Build history of the part. All positions in model axes, mm. A direction names the side the tool comes from. Coordinates: 2 decimals unless noted, no trailing zeros. Loops run counter-clockwise (first coordinate to the right, second up) from the corner with the lowest first, then second, coordinate; pieces in that order, holes last. Notation, with made-up numbers: (0, 89) - (57, 89) arc R16 cw to (57, 118) - close; hole circle Ø3 at (-22.75, 84.25). An arc over 180 degrees is marked (long way). One line per item, written item: value.
```python
from build123d import *

# Parameters (mm, degrees)
F1_DEPTH = 6.096
F3_DEPTH = 5.08
F4_W     = 19.05
F4_H     = 19.05
F5_DEPTH = 1.8542


with BuildPart() as f1:
    # F0 (on Top) → F1 (new body)
    with BuildSketch(Plane.XY):
        with BuildLine():
            ThreePointArc((0, 1.27), (0.371974, 0.371974), (1.27, 0))
            Line((1.27, 0), (15.24, 0))
            ThreePointArc((15.24, 0), (16.138026, 0.371974), (16.51, 1.27))
            Line((16.51, 1.27), (16.51, 15.24))
            ThreePointArc((16.51, 15.24), (16.138026, 16.138026), (15.24, 16.51))
            Line((15.24, 16.51), (1.27, 16.51))
            ThreePointArc((1.27, 16.51), (0.371974, 16.138026), (0, 15.24))
            Line((0, 15.24), (0, 1.27))
        make_face()
    extrude(amount=-F1_DEPTH)

    # F2 (on face) → F3 (cut)
    with BuildSketch(Plane(origin=(0, 0, -6.096), x_dir=(1, 0, 0), z_dir=(0, 0, -1))):
        with BuildLine():
            Line((13.97, -1.27), (2.54, -1.27))
            ThreePointArc((2.54, -1.27), (1.641974, -1.641974), (1.27, -2.54))
            Line((1.27, -2.54), (1.27, -13.97))
            ThreePointArc((1.27, -13.97), (1.641974, -14.868026), (2.54, -15.24))
            Line((2.54, -15.24), (13.97, -15.24))
            ThreePointArc((13.97, -15.24), (14.868026, -14.868026), (15.24, -13.97))
            Line((15.24, -13.97), (15.24, -2.54))
            ThreePointArc((15.24, -2.54), (14.868026, -1.641974), (13.97, -1.27))
        make_face()
    extrude(amount=-F3_DEPTH, mode=Mode.SUBTRACT)

    # F4 (on Top) → F5 (join)
    with BuildSketch(Plane.XY):
        with Locations((8.255, 8.255)):
            Rectangle(F4_W, F4_H)
    extrude(amount=F5_DEPTH)


solid = f1.part
```
Item 1: Tool access for faces 1 (the face through (0.382, 16.148, -3.005)), 2 (the face through (1.652, 1.632, -3.592)), 3 (the face through (16.148, 16.128, -3.005)): list every direction of +Z, -Z, +X, -X, +Y, -Y with a clear straight run to the whole face (end or side of a thin tool).
Check result:
face 1: -Z, -X, +Y
face 2: -Z
face 3: -Z, +X, +Y
Item 2: Drop flat-ended pins along their axis: P1, Ø2, axis at x = 13, z = -3, coming from the +Y side; P2, Ø3, axis at x = 11, z = -4.5, coming from the -Y side; P3, Ø4, axis at x = 9.5, y = 4, coming from the -Z side. Give the stop position or say it passes through.
Check result:
P1: stops at y = 16.51
P2: stops at y = 0
P3: stops at z = -1.02
Item 3: Cut at A-A, the plane z = -4.25. Write the cut outline in (x, y), then the cut area to 3 significant figures.
Check result:
outline: (0, 1.27) arc R1.27 ccw to (1.27, 0) - (15.24, 0) arc R1.27 ccw to (16.51, 1.27) - (16.51, 15.24) arc R1.27 ccw to (15.24, 16.51) - (1.27, 16.51) arc R1.27 ccw to (0, 15.24) - close; hole (1.27, 2.54) arc R1.27 ccw to (2.54, 1.27) - (13.97, 1.27) arc R1.27 ccw to (15.24, 2.54) - (15.24, 13.97) arc R1.27 ccw to (13.97, 15.24) - (2.54, 15.24) arc R1.27 ccw to (1.27, 13.97) - close
area: 77.4 mm^2
Item 4: Cut at B-B, the plane x = 11.75. Write the cut outline in (y, z), then the cut area to 3 significant figures.
Check result:
outline: (-1.27, 0) - (0, 0) - (0, -6.1) - (1.27, -6.1) - (1.27, -1.02) - (15.24, -1.02) - (15.24, -6.1) - (16.51, -6.1) - (16.51, 0) - (17.78, 0) - (17.78, 1.85) - (-1.27, 1.85) - close
area: 65.0 mm^2
Item 5: Probe probe 1 along Y at (x, z) = (4.5, -2.5); probe 2 along Z at (x, y) = (5.25, 6). List the from-to ranges inside material, lowest first. Write a range as from..to.
Check result:
probe 1: y = 0..1.27, 15.24..16.51
probe 2: z = -1.02..1.85
Item 6: Pull direction Y, two halves, no side cores. Call faces 4 (the face through (16.128, 0.362, -3.005)), 5 (the face through (8, 17.78, 1)), 6 (the face through (14.878, 1.652, -3.592)): released by +Y, released by -Y, zero draft, split by the parting line, or undercut.
Check result:
face 4: released by -Y
face 5: released by +Y
face 6: undercut
Item 7: Cut at D-D, the plane x = 1. Write the cut outline in (y, z), then the cut area to 3 significant figures.
Check result:
outline: (-1.27, 0) - (0.03, 0) - (0.03, -6.1) - (16.48, -6.1) - (16.48, 0) - (17.78, 0) - (17.78, 1.85) - (-1.27, 1.85) - close
area: 136 mm^2
